```python
from build123d import *

# Parameters (mm, degrees)
SKETCH1_R                = 3
SKETCH1_R_2              = 2
BOSS_EXTRUDE1_DEPTH      = 10
BOSS_EXTRUDE2_DEPTH      = 2
BOSS_EXTRUDE3_DEPTH      = 5
BOSS_EXTRUDE3_DEPTH_BACK = 5


with BuildPart() as part:
    # Sketch1 → Boss-Extrude1 (new body)
    with BuildSketch(Plane.XY):
        Circle(SKETCH1_R)
        Circle(SKETCH1_R_2, mode=Mode.SUBTRACT)
    extrude(amount=BOSS_EXTRUDE1_DEPTH)

    # Sketch2 → Boss-Extrude2 (add)
    with BuildSketch(Plane(origin=(0, 0, 0), x_dir=(-1, 0, 0), z_dir=(0, 0, -1))):
        Polygon((0, 5), (15, 5), (15, -5), (-15, -5), (-15, 5), align=None)
    extrude(amount=BOSS_EXTRUDE2_DEPTH)

    # Sketch4 → Boss-Extrude3 (add, two sides)
    with BuildSketch(Plane(origin=(0, 0, 0), x_dir=(1, 0, 0), z_dir=(0, 1, 0))) as boss_extrude3_sk:
        with BuildLine():
            ThreePointArc((-17, 17), (-14.577379737, 8.253572158), (-8, 2))
            Line((-8, 2), (-2.6e-08, 2))
            ThreePointArc((-2.6e-08, 2), (-10.606601727, 6.393398292), (-15, 17))
            Line((-15, 17), (-17, 17))
        make_face()
        with BuildLine():
            ThreePointArc((15, 17), (10.606601708, 6.393398273), (-2.6e-08, 2))
            Line((-2.6e-08, 2), (8, 2))
            ThreePointArc((8, 2), (14.577379737, 8.253572158), (17, 17))
            Line((17, 17), (15, 17))
        make_face()
    extrude(amount=BOSS_EXTRUDE3_DEPTH)
    extrude(boss_extrude3_sk.sketch, amount=-BOSS_EXTRUDE3_DEPTH_BACK)


solid = part.part
```
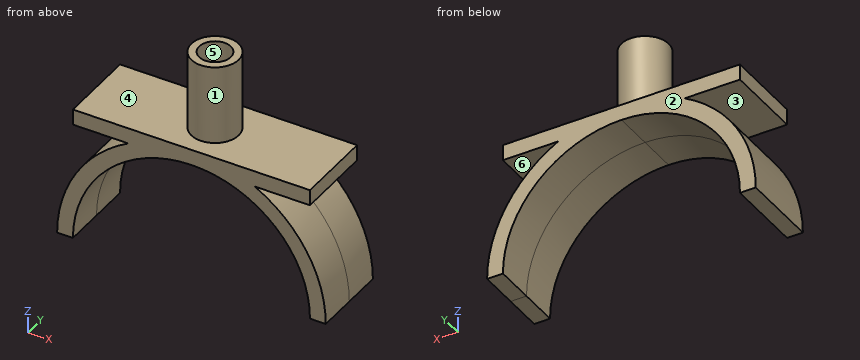
CAD build for the part. Positions are in the model's coordinates, mm. Face numbers are marked on the shaded views. A direction names the side the tool comes from. Coordinates: 2 decimals unless noted, no trailing zeros. Write each loop counter-clockwise with the first axis right and the second up, starting at its lowest first coordinate (ties: lowest second). Pieces come first, ordered by that corner, then holes.
(1) Two-plate mould, pull along Z, no slides. Class the marked faces 4, 5 and 6: +Z half, -Z half, draft (parallel to the pull), parting line (faces both ways), or undercut.
(2) Drill centre lines: probe 1 along Y at (x, z) = (0, 3); probe 2 along Z at (x, y) = (-12.5, -0.25); probe 3 along Z at (x, y) = (9, 4.75). Where is each one in solid material? Low to high.
(3) Cut at D-D, the plane z = 6. List the corners of the cut face in (x, y), and give its area (3 significant figures).
(4) Cut at A-A, the plane z = -3.5. List the corners of the cut face in (x, y).
(5) Flat gauge pins, fed straight in: pin 1 (3.5 mm diameter, centred on x = -11.5, y = 0, fed in from -Z); pin 2 (2 mm diameter, centred on x = 0, y = 0, fed in from +Z); pin 3 (1.6 mm diameter, centred on y = -2, z = -1.5, fed in from -X). Where does each tip first touch, or does it go through?
(6) Cut at C-C, the plane y = 0.75. List the corners of the cut face in (x, z), and give its area (3 significant figures).
(7) 3-axis set-ups, long thin cutter, end or side, ignore diameter. For the marked faces 1, 2 and 3: which of +Z, -Z, +X, -X, +Y, -Y reach the whole face in a straight line?
(8) Cut at B-B, the plane x = 14.5. List the corners of the cut face in (y, z).
Geometry says:
1. face 4: +Z half
1. face 5: draft
1. face 6: undercut
2. probe 1: y = -3 to -2, 2 to 3
2. probe 2: z = -8.71 to -5.48, -2 to 0
2. probe 3: z = -5 to -2.58, -2 to 0
3. outline: circle Ø6 at (0, 0); hole circle Ø4 at (0, 0)
3. area: 15.7 mm2
4. outline: (-10.33, -5) - (-6.54, -5) - (-6.54, 5) - (-10.33, 5) - close; (6.54, -5) - (10.33, -5) - (10.33, 5) - (6.54, 5) - close
5. pin 1: stops at z = -9.97
5. pin 2: stops at z = 0
5. pin 3: stops at x = -15
6. outline: (-17, -17) - (-15, -17) arc R15 cw to (15, -17) - (17, -17) arc R17 ccw to (8, -2) - (15, -2) - (15, 0) - (2.9, 0) - (2.9, 10) - (1.85, 10) - (1.85, 0) - (-1.85, 0) - (-1.85, 10) - (-2.9, 10) - (-2.9, 0) - (-15, 0) - (-15, -2) - (-8, -2) arc R17 ccw to start
6. area: 160 mm2
7. face 1: +Z
7. face 2: +Z, -Z, +X, -X, +Y
7. face 3: -X, +Y, -Y
8. outline: (-5, -13.16) - (5, -13.16) - (5, -8.13) - (-5, -8.13) - close; (-5, -2) - (5, -2) - (5, 0) - (-5, 0) - close
